Design review of the part built by this model. Coordinates are the model's own, in mm. Coordinates: 2 decimals unless noted, no trailing zeros. Write each loop counter-clockwise with the first axis right and the second up, starting at its lowest first coordinate (ties: lowest second). Pieces come first, ordered by that corner, then holes. Notation, with made-up numbers: (-1, 33.5) - (25, 33.5) arc R12 cw to (25, 42.5) - close; hole circle Ø2 at (-23.75, 50.25). An arc over 180 degrees is marked (long way). Use a Markdown table: item, result.
Solid Edge part; units mm, degrees
sketch "Sketch1" plane through (0, 0, 0) normal (0, 0, 1) x (1, 0, 0)
  line L0 (-165, -25) -> (165, -25)
  line L1 (165, -25) -> (165, 25)
  line L2 (165, 25) -> (-165, 25)
  line L3 (-165, 25) -> (-165, -25)
  dimension "D1" = 165
  dimension "D2" = 165
extrude "Protrusion1" add sketch "Sketch1" along normal blind 70
sketch "Sketch2" plane through (165, 0, 35) normal (1, 0, 0) x (0, 1, 0)
  line L0 (-25, 35) -> (7.5, -35)
  line L1 (7.5, -35) -> (25, -35)
  line L2 (25, -35) -> (25, -25)
  line L3 (12.8571, -25) -> (25, -25)
  line L4 (-15, 35) -> (12.8571, -25)
  line L5 (-25, 35) -> (-15, 35)
extrude "Extrusionsausschnitt_1" cut sketch "Sketch2" along normal mid plane 945.1558 flip side to cut
sketch "Sketch3" plane through (0, -111.4175, 35) normal (0, -1, 0) x (1, 0, 0)
  line L0 (-136.3397, 20) -> (-20, 20)
  line L1 (-20, 20) -> (-20, 15)
  line L2 (-20, 15) -> (-145, 15)
  line L3 (-145, 15) -> (-136.3397, 20)
  line L4 (-145, -5) -> (-20, -5)
  line L5 (-20, -5) -> (-20, -10)
  line L6 (-20, -10) -> (-136.3397, -10)
  line L7 (-136.3397, -10) -> (-145, -5)
  dimension "D1" = 145
  dimension "D2" = 145
  dimension "D3" = 136.3397
extrude "Extrusionsausschnitt_2" cut sketch "Sketch3" along normal mid plane 441.7858
mirror "Mirror1" about plane through (0, 0, 0) normal (1, 0, 0) of "Extrusionsausschnitt_2"
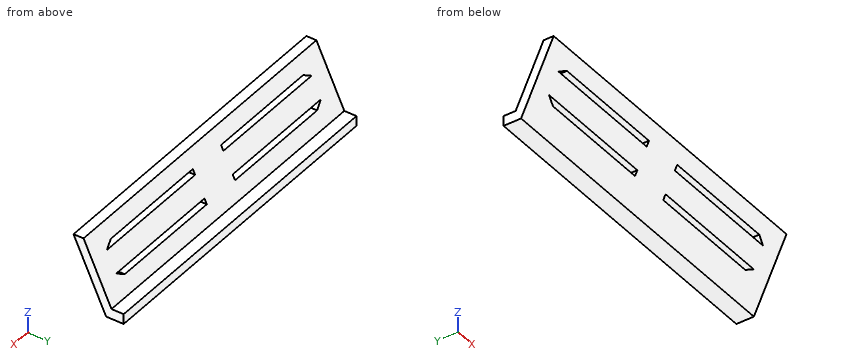
(1) Take a section at B-B on x = -1.5. Write out the cut boundary in (y, z), and give its area (3 significant figures).
Determined:
| item | result |
|---|---|
| outline | (-25, 70) - (7.5, 0) - (25, 0) - (25, 10) - (12.86, 10) - (-15, 70) - close |
| area | 798 mm2 |
(2) Take a section at C-C on z = 15. Write out the cut boundary in (x, y), and give its area (3 significant figures).
Determined:
| item | result |
|---|---|
| outline | (-165, 0.54) - (165, 0.54) - (165, 10.54) - (-165, 10.54) - close |
| area | 3,300 mm2 |
(3) Take a section at D-D on z = 39. Write out the cut boundary in (x, y).
Determined:
| item | result |
|---|---|
| outline | (-165, -10.61) - (165, -10.61) - (165, -0.61) - (-165, -0.61) - close |
(4) For L1, parallel to X at y = -9, z = 52; L2, parallel to Z at x = 81, y = -13; L3, parallel to Z at x = 62, y = 14.5, list the stretches that pass through material, from the lowest coordinate up. Write a range as from..to.
Determined:
| item | result |
|---|---|
| L1 | -165..-141.54, -20..20, 141.54..165 |
| L2 | 44.15..50, 55..65.69 |
| L3 | 0..10 |
(5) Take a section at A-A on x = 62.5. Write out the cut boundary in (y, z), and give its area (3 significant figures).
Determined:
| item | result |
|---|---|
| outline | (-25, 70) - (-18.04, 55) - (-8.04, 55) - (-15, 70) - close; (-15.71, 50) - (-6.43, 30) - (3.57, 30) - (-5.71, 50) - close; (-4.11, 25) - (7.5, 0) - (25, 0) - (25, 10) - (12.86, 10) - (5.89, 25) - close |
| area | 698 mm2 |
(6) For pin 1 (3 mm diameter, centred on x = 112.5, y = -11.5, fed in from +Z); pin 2 (5 mm diameter, centred on x = -105, y = -2.5, fed in from -Z); pin 3 (12 mm diameter, centred on x = 36, z = 34, fed in from -Y), all flat-tipped, find the tip position at first contact; note any pin that passes through.
Determined:
| item | result |
|---|---|
| pin 1 | z = 65.69 |
| pin 2 | z = 16.15 |
| pin 3 | y = -11.07 |
